```python
from build123d import *

# Parameters (mm, degrees)
PAD_DEPTH    = 4
SKETCH001_W  = 30
SKETCH001_H  = 8
PAD001_DEPTH = 6
POCKET_DEPTH = 1.6
CHAMFER_SIZE = 2
FILLET_R     = 1
PAD002_DEPTH = 4.4


with BuildPart() as part:
    # Sketch → Pad (new body)
    with BuildSketch(Plane.XY):
        with BuildLine():
            ThreePointArc((5, 29.999999), (0, 35), (-5, 29.999999))
            Line((-5, -5), (-5, 29.999999))
            Line((-15, -5), (-5, -5))
            Line((-15, -5), (-15, -13))
            Line((-15, -13), (15, -13))
            Line((15, -13), (15, -5))
            Line((5, -5), (15, -5))
            Line((5, 29.999999), (5, -5))
        make_face()
        with BuildLine():
            ThreePointArc((-1.6, 0), (0, -1.6), (1.6, 0))
            Line((1.6, 0), (1.6, 30))
            ThreePointArc((1.6, 30), (0, 31.6), (-1.6, 30))
            Line((-1.6, 0), (-1.6, 30))
        make_face(mode=Mode.SUBTRACT)
    extrude(amount=-PAD_DEPTH)

    # Sketch001 → Pad001 (join)
    with BuildSketch(Plane.XY):
        with Locations((0, -9)):
            Rectangle(SKETCH001_W, SKETCH001_H)
    extrude(amount=PAD001_DEPTH)

    # Sketch002 → Pocket (cut)
    with BuildSketch(Plane.XY.offset(6)):
        Polygon((-6, -10), (0, -16), (6, -10), (22.322094, -10), (22.322094, -1.337342), (-21.139692, -1.337342), (-21.139692, -10), align=None)
    extrude(amount=-POCKET_DEPTH, mode=Mode.SUBTRACT)

    # Chamfer
    chamfer_edges = [part.edges().sort_by_distance(p)[0] for p in [
        (15, -5, 2.2),
        (15, -13, 3),
        (-15, -5, 2.2),
        (-15, -13, 3),
    ]]
    chamfer(chamfer_edges, length=CHAMFER_SIZE)

    # Fillet
    fillet_edges = [part.edges().sort_by_distance(p)[0] for p in [
        (-6, -10, 5.2),
        (-3, -13, 5.2),
        (6, -10, 5.2),
        (3, -13, 5.2),
    ]]
    fillet(fillet_edges, radius=FILLET_R)

    # Sketch003 → Pad002 (join)
    with BuildSketch(Plane.XY):
        with BuildLine():
            ThreePointArc((5, 29.999992), (4e-06, 35), (-5, 30))
            Line((-5, 30), (-5, -5))
            Line((-5, -5), (5, -5))
            Line((5, -5), (5, 29.999992))
        make_face()
        Polygon((-2.75, -1.587713), (0, -3.175426), (2.75, -1.587713), (2.75, 31.587713), (0, 33.175426), (-2.75, 31.587713), align=None, mode=Mode.SUBTRACT)
    extrude(amount=PAD002_DEPTH)


solid = part.part
```
Can you work these out from the model? Positions are in its coordinate system, mm. A direction names the side the tool comes from. Round coordinates to 2 decimals unless told otherwise and drop trailing zeros. Order: outer loops, then holes, each group sorted by start corner. A loop starts at its lowest first (then second) coordinate and runs counter-clockwise, first axis right, second up. Notation, with made-up numbers: (-7, 84.25) -> (5, 84.25) arc R19 ccw to (5, 121.25) -> close; hole circle Ø3 at (9, 29.5). An arc over 180 degrees is marked (long way). Return JSON: item names as keys, results as strings. Group by question number.
1. Will these pins go through, and if not, where does the flat tip stop? pin 1 (5 mm diameter, centred on y = 24.5, z = -1.5, fed in from +X); pin 2 (4.5 mm diameter, centred on y = 19, z = -2, fed in from -X); pin 3 (0.8 mm diameter, centred on x = 9, z = 5, fed in from +Y); pin 4 (5 mm diameter, centred on x = -9, y = 17, fed in from +Z) (3 decimals).
2. If we section it at D-D, the plane z = 3.5: Write out the boundary of the cut face in (x, y).
3. If we section it at B-B, the plane z = -3: Write out the boundary of the cut face in (x, y), then the cut area to 3 significant figures.
4. If we section it at A-A, the plane y = 24.5: Write out the boundary of the cut face in (x, z), then the cut area to 3 significant figures.
5. Which directions (+Z, -Z, +X, -X, +Y, -Y) give clear straight access to the entire face, cutting with the end or side of a thin tool? Please do faces 1 (the face through (-1.6, 15, -2)), 2 (the face through (-2.75, 15, 2)), 3 (the face through (5, -11, 5)), 4 (the face through (5, 12, 0)).
6. We'd pull the mould along X, two halves only. Please class faces 5 (the face through (15, -9, 1)), 6 (the face through (-1.36, 32.39, 2.17)), 7 (the face through (-9, -5, 0)): released by +X, released by -X, zero draft, split by the parting line, or undercut.
7. If we section it at C-C, the plane x = 1: Write out the boundary of the cut face in (y, z).
8. I need wall thicknesses on line 1 (X direction, y = 1, z = -1.25); line 2 (X direction, y = 6.5, z = 3.5); line 3 (Y direction, x = -2, z = 3.25). Which ranges of each line are inside material? Lowest first, please. Write a range as [from, to].
Output values:
{
 "1": {"pin 1": "x = 5", "pin 2": "x = -5", "pin 3": "y = -10", "pin 4": "through"},
 "2": {"outline": "(-15, -11) -> (-13, -13) -> (13, -13) -> (15, -11) -> (15, -7) -> (13, -5) -> (5, -5) -> (5, 30) arc R5 ccw to (-5, 30) -> (-5, -5) -> (-13, -5) -> (-15, -7) -> close; hole (-2.75, -1.59) -> (0, -3.18) -> (2.75, -1.59) -> (2.75, 31.59) -> (0, 33.18) -> (-2.75, 31.59) -> close"},
 "3": {"outline": "(-15, -11) -> (-13, -13) -> (13, -13) -> (15, -11) -> (15, -7) -> (13, -5) -> (5, -5) -> (5, 30) arc R5 ccw to (-5, 30) -> (-5, -5) -> (-13, -5) -> (-15, -7) -> close; hole (-1.6, 0) arc R1.6 ccw to (1.6, 0) -> (1.6, 30) arc R1.6 ccw to (-1.6, 30) -> close", "area": "517 mm²"},
 "4": {"outline": "(-5, -4) -> (-1.6, -4) -> (-1.6, 0) -> (-2.75, 0) -> (-2.75, 4.4) -> (-5, 4.4) -> close; (1.6, -4) -> (5, -4) -> (5, 4.4) -> (2.75, 4.4) -> (2.75, 0) -> (1.6, 0) -> close", "area": "47.0 mm²"},
 "5": {"face 1": "+Z, -Z", "face 2": "+Z", "face 3": "+Z, +Y", "face 4": "+Z, -Z, +X, +Y"},
 "6": {"face 5": "released by +X", "face 6": "undercut", "face 7": "zero draft"},
 "7": {"outline": "(-13, -4) -> (-1.25, -4) -> (-1.25, 0) -> (-2.6, 0) -> (-2.6, 4.4) -> (-13, 4.4) -> close; (31.25, -4) -> (34.9, -4) -> (34.9, 4.4) -> (32.6, 4.4) -> (32.6, 0) -> (31.25, 0) -> close"},
 "8": {"line 1": "[-5, -1.6], [1.6, 5]", "line 2": "[-5, -2.75], [2.75, 5]", "line 3": "[-13, -2.02], [32.02, 34.58]"}
}
